Design review of the part shown in the three views and the two pictorial views. Dimensions are in mm from the part's minimum x, y and z. Coordinates: 2 decimals unless noted, no trailing zeros. Loops run counter-clockwise (first coordinate to the right, second up) from the corner with the lowest first, then second, coordinate; pieces in that order, holes last. Notation, with made-up numbers: (-2, -21) -> (26, -21) arc R8 ccw to (26, -6) -> close; hole circle Ø3 at (-22, 48). An arc over 180 degrees is marked (long way). Use CSV: the item, a comma, the result in double quotes.
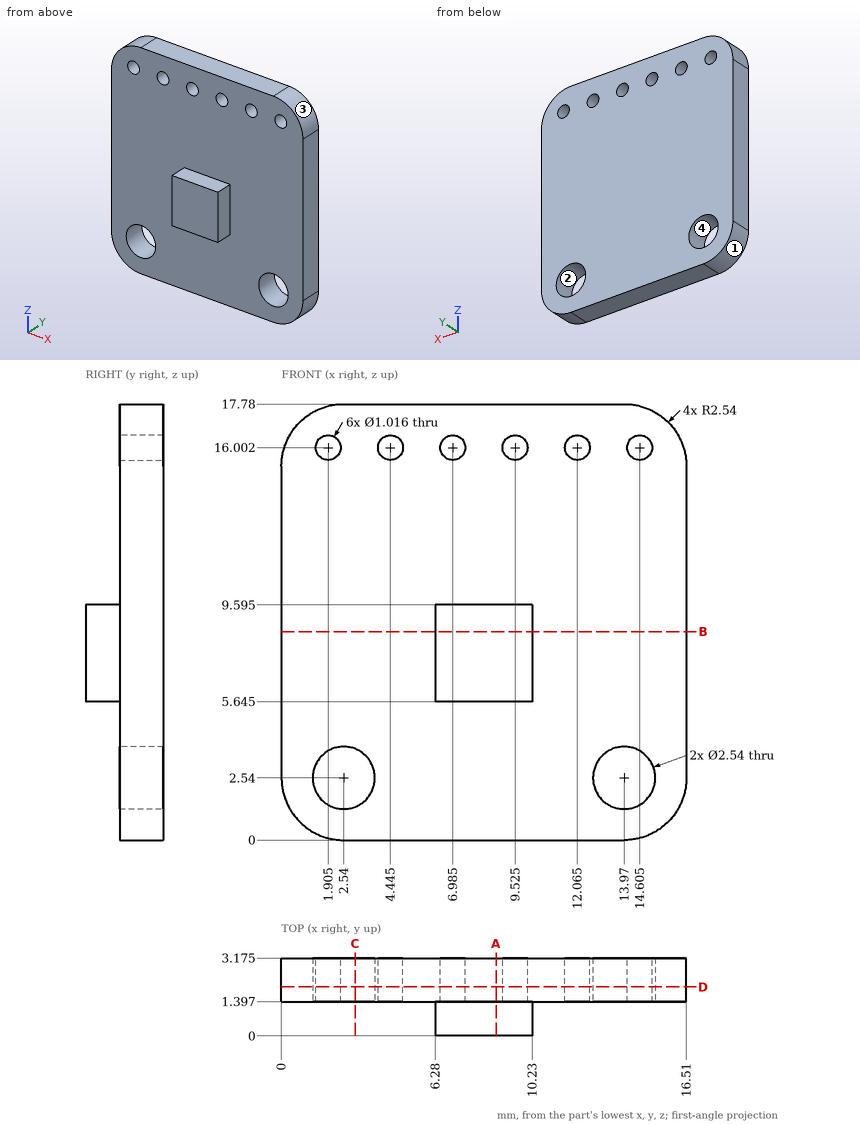
Item 1: Clearance check with flat-ended pins moving along their axes: pin 1 (3.5 mm diameter, centred on x = 2.54, z = 2.54, fed in from -Y); pin 2 (1.5 mm diameter, centred on x = 13.97, z = 2.54, fed in from -Y); pin 3 (1.1 mm diameter, centred on y = 0.5, z = 7.5, fed in from -X); pin 4 (1.1 mm diameter, centred on y = 0.5, z = 7.5, fed in from +X). State where each tip first meets the part, or that it passes through.
Checked values:
pin 1,"y = 1.4"
pin 2,"through"
pin 3,"x = 6.28"
pin 4,"x = 10.23"
Item 2: To check wall thickness, follow line 1 along X through (y, z) = (2, 2.54); line 2 along Z through (x, y) = (2.5, 1.85); line 3 along Z through (x, y) = (2.25, 2.35). State the ranges of each line that lie inside material, in increasing order.
Checked values:
line 1,"0 to 1.27, 3.81 to 12.7, 15.24 to 16.51"
line 2,"0 to 1.27, 3.81 to 17.78"
line 3,"0.02 to 1.3, 3.78 to 15.63, 16.37 to 17.76"
Item 3: Add section B-B (z = 8.5). Give the boundary of the cut face in (x, y) (3 decimals), then the cut area to 3 significant figures.
Checked values:
outline,"(0, 1.397) -> (6.28, 1.397) -> (6.28, 0) -> (10.23, 0) -> (10.23, 1.397) -> (16.51, 1.397) -> (16.51, 3.175) -> (0, 3.175) -> close"
area,"34.9 mm^2"
Item 4: Add section A-A (x = 8.75). Give the boundary of the cut face in (y, z) (3 decimals), then the cut area to 3 significant figures.
Checked values:
outline,"(0, 5.645) -> (1.397, 5.645) -> (1.397, 0) -> (3.175, 0) -> (3.175, 17.78) -> (1.397, 17.78) -> (1.397, 9.595) -> (0, 9.595) -> close"
area,"37.1 mm^2"
Item 5: Draft analysis for pull direction X (two halves, no side actions). For the marked faces 1, 2, 3 and 4, state which applies: pulls with the +X half, pulls with the -X half, needs draft (parallel to the pull), parting line crosses it, or undercut.
Checked values:
face 1,"pulls with the -X half"
face 2,"undercut"
face 3,"pulls with the +X half"
face 4,"undercut"
Item 6: Add section D-D (y = 2). State how many separate pieces and enclosed holes the cut face has, then the cut area to 3 significant figures.
Checked values:
separate pieces,"1"
enclosed holes,"8"
area,"273 mm^2"
Item 7: Add section C-C (x = 3). Give the boundary of the cut face in (y, z) (3 decimals).
Checked values:
outline,"(1.397, 0) -> (3.175, 0) -> (3.175, 1.356) -> (1.397, 1.356) -> close; (1.397, 3.724) -> (3.175, 3.724) -> (3.175, 17.78) -> (1.397, 17.78) -> close"
